Build history of the part. All positions in model axes, mm. Face numbers are marked on the shaded views. A direction names the side the tool comes from. Coordinates: 2 decimals unless noted, no trailing zeros. Order: outer loops, then holes, each group sorted by start corner. A loop starts at its lowest first (then second) coordinate and runs counter-clockwise, first axis right, second up. Notation, with made-up numbers: (43, -16.5) - (65, -16.5) arc R8 ccw to (65, -7.5) - close; hole circle Ø2 at (8.5, -23). An arc over 180 degrees is marked (long way). Write each question's results on one line, items separated by ' | '.
from build123d import *

# Parameters (mm, degrees)
F1_DEPTH = 20
F2_R     = 2.1
F3_DEPTH = 25


with BuildPart() as f1:
    # F0 (on Front) → F1 (new body)
    with BuildSketch(Plane.XZ):
        Polygon((0, 7.5), (0, 0), (2.5, 0), (2.5, 5), (5.7, 5), (5.7, -52), (19.7, -52), (19.7, -67), (22.2, -67), (22.2, -49.5), (8.2, -49.5), (8.2, 7.5), align=None)
    extrude(amount=F1_DEPTH)

    # F2 (on face) → F3 (join)
    with BuildSketch(Plane.YZ.offset(22.2)):
        with Locations((-10, -58.25)):
            Circle(F2_R)
    extrude(amount=F3_DEPTH)


solid = f1.part
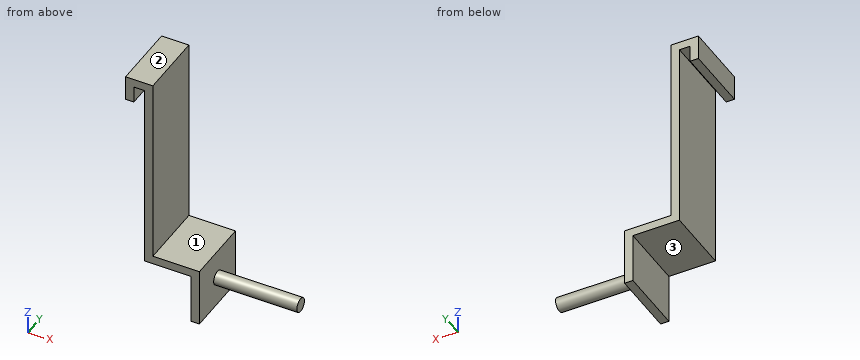
1. Band-saw the part on A-A on y = -10. Give the cut face in (x, z), then the cut area to 3 significant figures.
Solved:
outline: (0, 0) - (2.5, 0) - (2.5, 5) - (5.7, 5) - (5.7, -52) - (19.7, -52) - (19.7, -67) - (22.2, -67) - (22.2, -60.35) - (47.2, -60.35) - (47.2, -56.15) - (22.2, -56.15) - (22.2, -49.5) - (8.2, -49.5) - (8.2, 7.5) - (0, 7.5) - close | area: 353 mm2
2. Probe line 1 (Z direction, x = 44, y = -10); line 2 (Z direction, x = 8, y = -7.75); line 3 (X direction, y = -17.5, z = -44). List the from-to ranges inside material, lowest first.
Solved:
line 1: z = -60.35 to -56.15 | line 2: z = -52 to 7.5 | line 3: x = 5.7 to 8.2
3. Drop flat-ended pins along their axis: pin 1 Ø7.5 at (y, z) = (-9.5, -58) entering from -X; pin 2 Ø1.5 at (x, y) = (20, -14) entering from +Z; pin 3 Ø7 at (x, y) = (14, -6.5) entering from -Z; pin 4 Ø1.5 at (x, y) = (40, -7) entering from +Z. Give the stop position or say it passes through.
Solved:
pin 1: stops at x = 19.7 | pin 2: stops at z = -49.5 | pin 3: stops at z = -52 | pin 4: passes through
4. Band-saw the part on B-B on z = -58.25. Give the cut face in (x, y), then the cut area to 3 significant figures.
Solved:
outline: (19.7, -20) - (22.2, -20) - (22.2, -12.1) - (47.2, -12.1) - (47.2, -7.9) - (22.2, -7.9) - (22.2, 0) - (19.7, 0) - close | area: 155 mm2
5. Band-saw the part on D-D on y = -2.75. Give the cut face in (x, z), then the cut area to 3 significant figures.
Solved:
outline: (0, 0) - (2.5, 0) - (2.5, 5) - (5.7, 5) - (5.7, -52) - (19.7, -52) - (19.7, -67) - (22.2, -67) - (22.2, -49.5) - (8.2, -49.5) - (8.2, 7.5) - (0, 7.5) - close | area: 248 mm2
6. Tool access for the marked faces 1, 2 and 3: list every direction of +Z, -Z, +X, -X, +Y, -Y with a clear straight run to the whole face (end or side of a thin tool).
Solved:
face 1: +Z, +X, +Y, -Y | face 2: +Z, +X, -X, +Y, -Y | face 3: -Z, -X, +Y, -Y
7. Band-saw the part on C-C on x = 10. Give the cut face in (y, z), then the cut area to 3 significant figures.
Solved:
outline: (-20, -52) - (0, -52) - (0, -49.5) - (-20, -49.5) - close | area: 50.0 mm2
